from build123d import *

# Parameters (mm, degrees)
SKETCH_1_R      = 1.6
EXTRUDE_1_DEPTH = 2
SKETCH_2_W      = 60
SKETCH_2_H      = 1.5
EXTRUDE_2_DEPTH = 50
FILLET_1_R      = 1


with BuildPart() as part:
    # 草图1 → 凸台-拉伸1 (new body)
    with BuildSketch(Plane.XY):
        Polygon((15, 0), (75, 0), (75, -8.5), (0, -8.5), (0, -1.5), (15, -1.5), align=None)
        with Locations((10, -5)):
            Circle(SKETCH_1_R, mode=Mode.SUBTRACT)
        with Locations((60, -5)):
            Circle(SKETCH_1_R, mode=Mode.SUBTRACT)
    extrude(amount=EXTRUDE_1_DEPTH)

    # 草图2 → 凸台-拉伸2 (add)
    with BuildSketch(Plane.XY.offset(2)):
        with Locations((45, -0.75)):
            Rectangle(SKETCH_2_W, SKETCH_2_H)
    extrude(amount=EXTRUDE_2_DEPTH)

    # 圆角1
    fillet_1_edges = [part.edges().sort_by_distance(p)[0] for p in [
        (75, -8.5, 1),
        (0, -8.5, 1),
        (45, -1.5, 2),
        (15, -0.75, 52),
        (75, -0.75, 52),
        (45, 0, 0),
    ]]
    fillet(fillet_1_edges, radius=FILLET_1_R)


solid = part.part
Check sheet for the modelled part. Datum: model origin and axes. Units: mm. A direction names the side the tool comes from. Round coordinates to 2 decimals unless told otherwise and drop trailing zeros. Loops run counter-clockwise (first coordinate to the right, second up) from the corner with the lowest first, then second, coordinate; pieces in that order, holes last.
1. Sectioned sample at C-C on x = 63. Record the boundary of the cut face in (y, z), and give its area (3 significant figures).
2. Set-up check for faces 5 (the flat face through (7, -1.5, 1)), 6 (the flat face through (0, -5, 1)), 7 (the flat face through (45, -1.5, 27)): record each of +Z, -Z, +X, -X, +Y, -Y from which the full face is reachable in a straight line by a thin tool's end or side.
3. Scan lines: probe 1 along Y at (x, z) = (10, 1.4); probe 2 along Y at (x, z) = (60, 1); probe 3 along Y at (x, z) = (66, 47). Record each from-to range of solid material in increasing order.
4. Sectioned sample at A-A on x = 10. Record the boundary of the cut face in (y, z), and give its area (3 significant figures).
5. Sectioned sample at B-B on y = -5. Record the boundary of the cut face in (x, z), and give its area (3 significant figures).
6. Gauge pin test, flat ends, axial feed: pin 1 Ø1 at (x, z) = (9, 1.5) entering from +Y; pin 2 Ø2 at (x, y) = (9.5, -1.5) entering from +Z; pin 3 Ø24.5 at (x, z) = (60, 18) entering from -Y; pin 4 Ø5 at (y, z) = (-6, 33.5) entering from +X. Record the tip position at first contact, or that the pin passes through.
7. Mould release check, pull along Y, two halves, no side actions. Record for faces 1 (the cylindrical face through (8.4, -4.93, 0.99)), 2 (the flat face through (38, -8.5, 1)), 3 (the flat face through (15, -1, 25)), 4 (the cylindrical face through (61.526, -4.519, 0.986)): released by +Y, released by -Y, zero draft, split by the parting line, or undercut.
8. Sectioned sample at D-D on z = 24. Record the boundary of the cut face in (x, y).
Recorded:
1. outline: (-8.5, 0) - (-1, 0) arc R1 ccw to (0, 1) - (0, 52) - (-1.5, 52) - (-1.5, 3) arc R1 cw to (-2.5, 2) - (-8.5, 2) - close
1. area: 92.0 mm2
2. face 5: +Z, -Z, -X, +Y
2. face 6: +Z, -Z, -X, +Y, -Y
2. face 7: +Z, +X, -X, -Y
3. probe 1: y = -8.5 to -6.6, -3.4 to -1.5
3. probe 2: y = -8.5 to -6.6, -3.4 to 0
3. probe 3: y = -1.5 to 0
4. outline: (-8.5, 0) - (-6.6, 0) - (-6.6, 2) - (-8.5, 2) - close; (-3.4, 0) - (-1.5, 0) - (-1.5, 2) - (-3.4, 2) - close
4. area: 7.60 mm2
5. outline: (0, 0) - (8.4, 0) - (8.4, 2) - (0, 2) - close; (11.6, 0) - (58.4, 0) - (58.4, 2) - (11.6, 2) - close; (61.6, 0) - (75, 0) - (75, 2) - (61.6, 2) - close
5. area: 137 mm2
6. pin 1: stops at y = -1.5
6. pin 2: stops at z = 2
6. pin 3: stops at y = -1.5
6. pin 4: passes through
7. face 1: undercut
7. face 2: released by -Y
7. face 3: zero draft
7. face 4: undercut
8. outline: (15, -1.5) - (75, -1.5) - (75, 0) - (15, 0) - close
